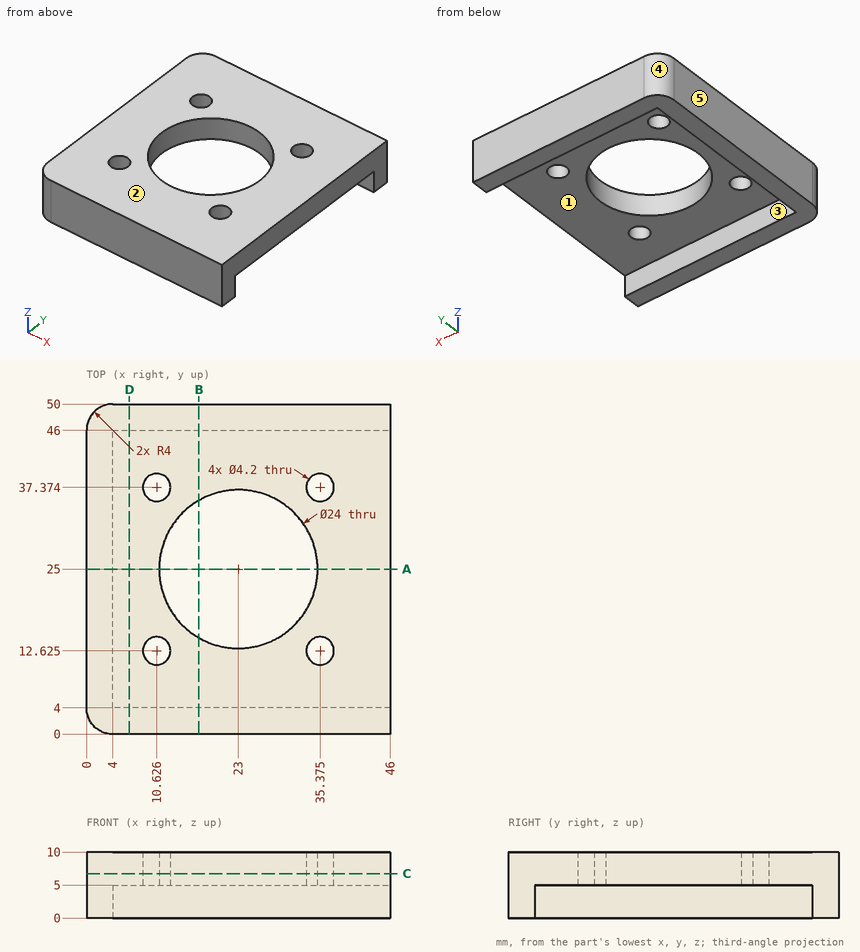
Could you check a few things on this drawing? It's one solid part, dimensions in mm from its lowest x, y, z. A direction names the side the tool comes from. Coordinates: 2 decimals unless noted, no trailing zeros. Write each loop counter-clockwise with the first axis right and the second up, starting at its lowest first coordinate (ties: lowest second). Pieces come first, ordered by that corner, then holes.
1) I'm going to push a flat-ended pin straight in: pin 1 (5.5 mm diameter, centred on x = 35.37, y = 12.63, fed in from -Z). Where does the tip first touch, or does it pass through?
Filled in:
pin 1: stops at z = 5
2) If we section it at B-B (x = 17): List the corners of the cut face in (y, z) for me.
Filled in:
outline: (0, 0) - (4, 0) - (4, 5) - (14.61, 5) - (14.61, 10) - (0, 10) - close; (35.39, 5) - (46, 5) - (46, 0) - (50, 0) - (50, 10) - (35.39, 10) - close
3) Thinking about a two-plate mould opening in Y: for the marked faces 3, 4 and 5, which applies, +Y half, -Y half, draft (parallel to the pull), parting line (faces both ways), or undercut?
Filled in:
face 3: undercut
face 4: +Y half
face 5: draft
4) If we section it at D-D (x = 6.5): List the corners of the cut face in (y, z) for me, plus the area to 3 significant figures.
Filled in:
outline: (0, 0) - (4, 0) - (4, 5) - (46, 5) - (46, 0) - (50, 0) - (50, 10) - (0, 10) - close
area: 290 mm2
5) If we section it at C-C (z = 6.75): List the corners of the cut face in (x, y) for me (1 decimal), plus the area to 3 significant figures.
Filled in:
outline: (0, 4) arc R4 ccw to (4, 0) - (46, 0) - (46, 50) - (4, 50) arc R4 ccw to (0, 46) - close; hole circle Ø4.2 at (10.6, 12.6); hole circle Ø4.2 at (10.6, 37.4); hole circle Ø24 at (23, 25); hole circle Ø4.2 at (35.4, 12.6); hole circle Ø4.2 at (35.4, 37.4)
area: 1,790 mm2
6) Which directions (+Z, -Z, +X, -X, +Y, -Y) give clear straight access to the entire face, cutting with the end or side of a thin tool? Please do the marked faces 1 and 2.
Filled in:
face 1: -Z, +X
face 2: +Z, +X, -X, +Y, -Y
7) If I drill on line 1 (Y direction, x = 4.5, z = 3.5); line 2 (Y direction, x = 23, z = 8.55); line 3 (X direction, y = 10.5, z = 1.5), over which ranges is the centre line in solid material (lowest first)?
Filled in:
line 1: y = 0 to 4, 46 to 50
line 2: y = 0 to 13, 37 to 50
line 3: x = 0 to 4
8) If we section it at A-A (y = 25): List the corners of the cut face in (x, z) for me, plus the area to 3 significant figures.
Filled in:
outline: (0, 0) - (4, 0) - (4, 5) - (11, 5) - (11, 10) - (0, 10) - close; (35, 5) - (46, 5) - (46, 10) - (35, 10) - close
area: 130 mm2
